Autodesk Inventor part; units mm, degrees
ref_plane "YZ Plane" through (0, 0, 0) normal (1, 0, 0) x (0, 1, 0)
ref_plane "XZ Plane" through (0, 0, 0) normal (0, 1, 0) x (-1, 0, 0)
ref_plane "XY Plane" through (0, 0, 0) normal (0, 0, 1) x (1, 0, 0)
sketch "草图1" plane through (0, 0, 0) normal (0, 0, 1) x (1, 0, 0)
  circle A0 centre (0, 0) radius 20
  circle A1 centre (0, 0) radius 10
  point P0 (0, 0)
extrude "拉伸1" add sketch "草图1" along normal blind 40 contours A0 | A1
sketch "草图2" plane through (0, 0, 40) normal (0, 0, 1) x (1, 0, 0)
  circle A0 centre (0, 0) radius 20
  point P0 (0, 0)
extrude "拉伸2" add sketch "草图2" along normal blind 50
sketch "草图3" plane through (0, 0, 90) normal (0, 0, 1) x (1, 0, 0)
  line L0 (0, 0) -> (0, 22.0262)
  line L1 (-10.5, -7.5) -> (-14.5, -7.5)
  line L2 (-14.5, -7.5) -> (-14.5, 7.5)
  line L3 (-14.5, 7.5) -> (-10.5, 7.5)
  line L4 (-10.5, 7.5) -> (-10.5, -7.5)
  line L5 (-10.5, -7.5) -> (-14.5, 7.5) construction
  line L6 (-14.5, -7.5) -> (-10.5, 7.5) construction
  line L7 (10.5, -7.5) -> (14.5, -7.5)
  line L8 (14.5, -7.5) -> (14.5, 7.5)
  line L9 (14.5, 7.5) -> (10.5, 7.5)
  line L10 (10.5, 7.5) -> (10.5, -7.5)
  line L11 (10.5, -7.5) -> (14.5, 7.5) construction
  line L12 (14.5, -7.5) -> (10.5, 7.5) construction
  point P0 (-12.5, 0)
  point P1 (12.5, 0)
  point P2 (-12.5, 0)
  dimension "d4" = 25
  dimension "d5" = 4
  dimension "d6" = 15
extrude "拉伸3" add sketch "草图3" along normal blind 45
full round fillet "全圆角1" first side at (-13.1667, -7.5, 105) centre faces at (-11.8333, -2.5, 135) second side at (-11.8333, 7.5, 105)
full round fillet "全圆角2" first side at (13.1667, 7.5, 105) centre faces at (13.1667, -2.5, 135) second side at (11.8333, -7.5, 105)
sketch "草图4" plane through (-14.5, -7.5, 90) normal (-1, 0, 0) x (0, 0, 1)
  arc A0 (37.5, 0) -> (37.5, 15) centre (37.5, 7.5) ccw
  point P0 (-90, 7.5)
hole "孔1" at (-14.5, 0, 127.5) direction (1, 0, 0) diameter 8 end through all
sketch "草图5" plane through (0, 0, 0) normal (0, 0, -1) x (-1, 0, 0)
  circle A0 centre (0, 0) radius 20
  point P0 (0, 0)
hole "孔2" at (0, 0, 0) direction (0, 0, 1) diameter 20 depth 40
properties part number "节块"
Could you check a few things on this model? Use its own coordinates, in mm. A direction names the side the tool comes from. Coordinates: 2 decimals unless noted, no trailing zeros. Order: outer loops, then holes, each group sorted by start corner. A loop starts at its lowest first (then second) coordinate and runs counter-clockwise, first axis right, second up. Notation, with made-up numbers: (45, -26.5) -> (54, -26.5) arc R22 cw to (54, -8.5) -> close; hole circle Ø11 at (26.25, -8.75). An arc over 180 degrees is marked (long way). One line per item, written item: value. Start each with the question number.
1) Which directions (+Z, -Z, +X, -X, +Y, -Y) give clear straight access to the entire face, cutting with the end or side of a thin tool? Please do faces 1 (the flat face through (12, -7.5, 108)), 2 (the flat face through (10.5, 0, 112)), 3 (the flat face through (0, 0, 40)).
2) Imagine slicing it at C-C on x = 0. List the corners of the cut face in (y, z) for me, plus the area to 3 significant figures.
3) I'm going to push flat-ended pins straight in: pin 1 (4.5 mm diameter, centred on x = -11.5, z = 107.5, fed in from +Y); pin 2 (9 mm diameter, centred on y = 0, z = 127.5, fed in from -X); pin 3 (2 mm diameter, centred on x = 0, z = 18, fed in from +Y). Where does each tip first touch, or does it pass through?
4) Imagine slicing it at D-D on z = 27.5. List the corners of the cut face in (x, y) for me, plus the area to 3 significant figures.
5) We'd pull the mould along Y, two halves only. Please class faces 4 (the flat face through (14.5, 0, 112)), 5 (the cylindrical face through (-12.472, -0.176, 123.504)), 6 (the flat face through (13, 7.5, 108)): +Y half, -Y half, draft (parallel to the pull), parting line (faces both ways), or undercut.
6) Imagine slicing it at B-B on z = 115.5. List the corners of the cut face in (x, y) for me, plus the area to 3 significant figures.
7) If I drill on L1, parallel to Y at x = -11.4, z = 127.5; L2, parallel to X at y = 6, z = 124; L3, parallel to Z at x = 11.6, y = 0, over which ranges is the centre line in solid material (lowest first)? Write a range as [from, to].
Answer list:
1. face 1: +Z, +X, -X, -Y
1. face 2: +Z, +Y, -Y
1. face 3: -Z
2. outline: (-20, 0) -> (-10, 0) -> (-10, 40) -> (10, 40) -> (10, 0) -> (20, 0) -> (20, 90) -> (-20, 90) -> close
2. area: 2,800 mm2
3. pin 1: stops at y = 7.5
3. pin 2: stops at x = -14.5
3. pin 3: stops at y = 20
4. outline: circle Ø40 at (0, 0); hole circle Ø20 at (0, 0)
4. area: 942 mm2
5. face 4: draft
5. face 5: undercut
5. face 6: +Y half
6. outline: (-14.5, -7.5) -> (-10.5, -7.5) -> (-10.5, 7.5) -> (-14.5, 7.5) -> close; (10.5, -7.5) -> (14.5, -7.5) -> (14.5, 7.5) -> (10.5, 7.5) -> close
6. area: 120 mm2
7. L1: y = [-7.5, -4], [4, 7.5]
7. L2: x = [-14.5, -10.5], [10.5, 14.5]
7. L3: z = [0, 123.5], [131.5, 135]
